from build123d import *

# Parameters (mm, degrees)
SKETCH1_W                     = 50.8
SKETCH1_H                     = 50.8
SKETCH1_W_2                   = 47.6
SKETCH1_H_2                   = 47.6
BOSS_EXTRUDE1_DEPTH           = 180
SKETCH6_R                     = 7.5
SKETCH6_R_2                   = 8
CUT_EXTRUDE1_DEPTH            = 189.747980122
M4_CLEARANCE_HOLE1_AT_2_COUNT = 2
M4_CLEARANCE_HOLE1_AT_2_PITCH = 20.8
CIRPATTERN1_COUNT             = 4
M5_CLEARANCE_HOLE1_D          = 5.5
M5_CLEARANCE_HOLE1_DEPTH      = 19.75
M5_CLEARANCE_HOLE1_TIP        = 1.652366702
CUT_EXTRUDE2_DEPTH            = 1.6
CUT_EXTRUDE3_DEPTH            = 1.6


with BuildPart() as part:
    # Sketch1 → Boss-Extrude1 (new body)
    with BuildSketch(Plane.XY):
        Rectangle(SKETCH1_W, SKETCH1_H)
        Rectangle(SKETCH1_W_2, SKETCH1_H_2, mode=Mode.SUBTRACT)
    extrude(amount=BOSS_EXTRUDE1_DEPTH)

    # Sketch6 → Cut-Extrude1 (cut, through all)
    with BuildSketch(Plane(origin=(0, 25.4, 0), x_dir=(1, 0, 0), z_dir=(0, 1, 0))):
        with Locations(Location((0, -160, 0), (0, 0, 270))):
            Circle(SKETCH6_R)
        with Locations(Location((0, -110, 0), (0, 0, 270))):
            Circle(SKETCH6_R_2)
    extrude(amount=-CUT_EXTRUDE1_DEPTH, mode=Mode.SUBTRACT)

    # Sketch8 → M4 Clearance Hole1 (revolve, cut)
    with BuildSketch(Plane(origin=(-25.4, -10.4, 7), x_dir=(0, 0, 1), z_dir=(0, 1, 0))):
        Polygon((0, 0), (0, 12.851936393), (2.25, 11.5), (2.25, 0), align=None)
    m4_clearance_hole1 = revolve(axis=Axis((-31.75, -10.4, 7), (1, 0, 0)), mode=Mode.SUBTRACT)

    # M4 Clearance Hole1 at 2: M4 Clearance Hole1 ×2
    with Locations(*[(0, i * M4_CLEARANCE_HOLE1_AT_2_PITCH, 0) for i in range(1, M4_CLEARANCE_HOLE1_AT_2_COUNT)]):
        add(m4_clearance_hole1, mode=Mode.SUBTRACT)

    # CirPattern1: M4 Clearance Hole1 ×4 about axis
    cirpattern1_axis = Axis((0, 0, 0), (0, 0, 1))
    for i in range(1, CIRPATTERN1_COUNT):
        add(m4_clearance_hole1.rotate(cirpattern1_axis, i * 360 / CIRPATTERN1_COUNT), mode=Mode.SUBTRACT)

    # CirPattern1 copy 1 sketch → CirPattern1 copy 1 (revolve, cut)
    with BuildSketch(Plane(origin=(-10.4, -25.4, 7), x_dir=(0, 0, 1), z_dir=(-1, 0, 0))):
        Polygon((0, 0), (0, 12.851936393), (2.25, 11.5), (2.25, 0), align=None)
    revolve(axis=Axis((-10.4, -31.75, 7), (0, 1, 0)), mode=Mode.SUBTRACT)

    # CirPattern1 copy 2 sketch → CirPattern1 copy 2 (revolve, cut)
    with BuildSketch(Plane(origin=(25.4, -10.4, 7), x_dir=(0, 0, 1), z_dir=(0, -1, 0))):
        Polygon((0, 0), (0, 12.851936393), (2.25, 11.5), (2.25, 0), align=None)
    revolve(axis=Axis((31.75, -10.4, 7), (-1, 0, 0)), mode=Mode.SUBTRACT)

    # CirPattern1 copy 3 sketch → CirPattern1 copy 3 (revolve, cut)
    with BuildSketch(Plane(origin=(10.4, 25.4, 7), x_dir=(0, 0, 1), z_dir=(1, 0, 0))):
        Polygon((0, 0), (0, 12.851936393), (2.25, 11.5), (2.25, 0), align=None)
    revolve(axis=Axis((10.4, 31.75, 7), (0, -1, 0)), mode=Mode.SUBTRACT)

    # M5 Clearance Hole1
    with Locations(Plane.XZ.offset(25.4)):
        with Locations((15, 140), (-15, 140), (-15, 45.7), (15, 45.7)):
            Hole(M5_CLEARANCE_HOLE1_D / 2, depth=M5_CLEARANCE_HOLE1_DEPTH)
            with Locations((0, 0, -(M5_CLEARANCE_HOLE1_DEPTH + M5_CLEARANCE_HOLE1_TIP / 2))):  # 118° drill point
                Cone(0, M5_CLEARANCE_HOLE1_D / 2, M5_CLEARANCE_HOLE1_TIP, mode=Mode.SUBTRACT)

    # Sketch13 → Cut-Extrude2 (cut)
    with BuildSketch(Plane(origin=(0, -25.4, 0), x_dir=(-1, 0, 0), z_dir=(0, -1, 0))):
        with BuildLine():
            Line((-13, -93), (-25.4, -93))
            ThreePointArc((-25.4, -93), (-28.4, -90), (-25.4, -87))
            Line((-25.4, -87), (-13, -87))
            ThreePointArc((-13, -87), (-10, -90), (-13, -93))
        make_face()
    extrude(amount=-CUT_EXTRUDE2_DEPTH, mode=Mode.SUBTRACT)

    # Sketch14 → Cut-Extrude3 (cut)
    with BuildSketch(Plane(origin=(25.4, 0, 0), x_dir=(0, 0, -1), z_dir=(1, 0, 0))):
        with BuildLine():
            Line((-97, -17.8), (-83, -17.8))
            ThreePointArc((-83, -17.8), (-80, -20.8), (-83, -23.8))
            Line((-83, -23.8), (-97, -23.8))
            ThreePointArc((-97, -23.8), (-100, -20.8), (-97, -17.8))
        make_face()
    extrude(amount=-CUT_EXTRUDE3_DEPTH, mode=Mode.SUBTRACT)


solid = part.part
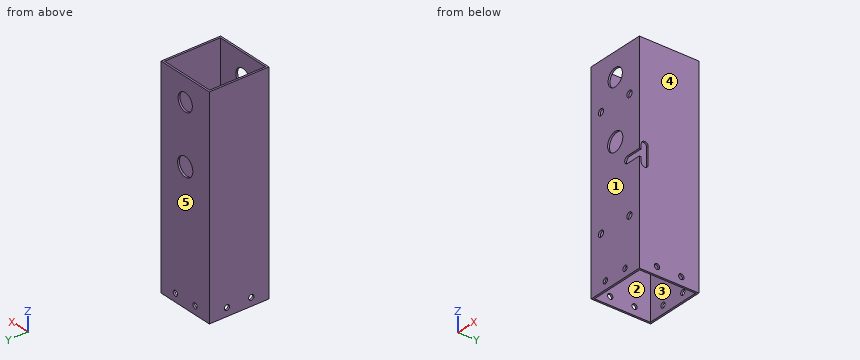
The listing builds one solid part. Answer for the finished solid, in the listing's coordinates (mm). Face numbers are marked on the shaded views. A direction names the side the tool comes from. Round coordinates to 2 decimals unless told otherwise and drop trailing zeros. Loops run counter-clockwise (first coordinate to the right, second up) from the corner with the lowest first, then second, coordinate; pieces in that order, holes last. Notation, with made-up numbers: M 29,-32.75 L 46,-32.75 A22 ccw 46,-7.75 Z; hole C 1,34 d6. An arc over 180 degrees is marked long. Return JSON: item names as keys, results as strings.
Q1. Each of these flat-tipped pins is pushed along its axis until it touches: pin 1 Ø6.5 at (x, z) = (15, 45.7) entering from -Y; pin 2 Ø4.5 at (x, z) = (15, 140) entering from -Y. Where does it stop, or does it pass through?
Results list:
{"pin 1": "stops at y = -25.4", "pin 2": "stops at y = 23.8"}
Q2. Find section B-B, the plane x = 20. Determine the outline of the cut face in (y, z), plus the area to 3 significant figures.
Results list:
{"outline": "M -25.4,0 L -23.8,0 L -23.8,87 L -25.4,87 Z; M -25.4,93 L -23.8,93 L -23.8,180 L -25.4,180 Z; M 23.8,0 L 25.4,0 L 25.4,180 L 23.8,180 Z", "area": "566 mm2"}
Q3. The mould has two halves that part along Y. Classify the marked faces 3, 4 and 5: released by +Y, released by -Y, zero draft, split by the parting line, or undercut.
Results list:
{"face 3": "undercut", "face 4": "zero draft", "face 5": "released by +Y"}
Q4. Find the intervals of material crossed by line 1 along X through (y, z) = (-24.8, 140); line 2 along Z through (x, y) = (-15, -24.25); line 3 along X through (y, z) = (17, 12), in increasing order. Write a range as from..to.
Results list:
{"line 1": "x = -25.4..-17.75, -12.25..12.25, 17.75..25.4", "line 2": "z = 0..42.95, 48.45..137.25, 142.75..180", "line 3": "x = -25.4..-23.8, 23.8..25.4"}
Q5. Which of the six approach directions +Z, -Z, +X, -X, +Y, -Y give full straight-line access (tool end or side, diameter ignored) to the marked faces 1 and 2?
Results list:
{"face 1": "+Z, -Z, +X, -X, -Y", "face 2": "+Z, -Z"}
Q6. Find section D-D, the plane y = -20.8. Determine the outline of the cut face in (x, z), plus the area to 3 significant figures.
Results list:
{"outline": "M -25.4,0 L -23.8,0 L -23.8,180 L -25.4,180 Z; M 23.8,0 L 25.4,0 L 25.4,80 L 23.8,80 Z; M 23.8,100 L 25.4,100 L 25.4,180 L 23.8,180 Z", "area": "544 mm2"}
Q7. Find section A-A, the plane x = 0. Determine the outline of the cut face in (y, z).
Results list:
{"outline": "M -25.4,0 L -23.8,0 L -23.8,102 L -25.4,102 Z; M -25.4,118 L -23.8,118 L -23.8,152.5 L -25.4,152.5 Z; M -25.4,167.5 L -23.8,167.5 L -23.8,180 L -25.4,180 Z; M 23.8,0 L 25.4,0 L 25.4,102 L 23.8,102 Z; M 23.8,118 L 25.4,118 L 25.4,152.5 L 23.8,152.5 Z; M 23.8,167.5 L 25.4,167.5 L 25.4,180 L 23.8,180 Z"}
Q8. Find section C-C, the plane z = 110. Determine the outline of the cut face in (x, y).
Results list:
{"outline": "M -25.4,-25.4 L -8,-25.4 L -8,-23.8 L -23.8,-23.8 L -23.8,23.8 L -8,23.8 L -8,25.4 L -25.4,25.4 Z; M 8,-25.4 L 25.4,-25.4 L 25.4,25.4 L 8,25.4 L 8,23.8 L 23.8,23.8 L 23.8,-23.8 L 8,-23.8 Z"}
